```python
from build123d import *

# Parameters (mm, degrees)
SKETCH1_R           = 11
BOSS_EXTRUDE1_DEPTH = 20.45
SKETCH2_R           = 11
SKETCH2_R_2         = 10.8
CUT_EXTRUDE1_DEPTH  = 30.5
SKETCH5_R           = 0.8
CUT_EXTRUDE2_DEPTH  = 3
BOSS_EXTRUDE2_DEPTH = 2
SKETCH7_R           = 3
BOSS_EXTRUDE3_DEPTH = 12
CUT_EXTRUDE3_DEPTH  = 1
CIRPATTERN1_COUNT   = 4
CIRPATTERN2_COUNT   = 4
SKETCH11_R          = 5
BOSS_EXTRUDE4_DEPTH = 0.25
SKETCH12_R          = 11.05
BOSS_EXTRUDE5_DEPTH = 7
SKETCH14_R          = 1.0375
CUT_EXTRUDE4_DEPTH  = 3
SKETCH16_R          = 10.8
SKETCH16_R_2        = 10.3
CUT_EXTRUDE5_DEPTH  = 1.5
CUT_EXTRUDE6_DEPTH  = 0.5
CUT_EXTRUDE7_DEPTH  = 1.5
CHAMFER1_SIZE       = 0.25
CUT_EXTRUDE8_DEPTH  = 0.5
SKETCH20_R          = 0.5
BOSS_EXTRUDE7_DEPTH = 0.5
CIRPATTERN4_COUNT   = 2
SKETCH22_R          = 3
BOSS_EXTRUDE8_DEPTH = 2
SKETCH23_R          = 1
BOSS_EXTRUDE9_DEPTH = 9.2
CHAMFER2_SIZE       = 0.25
SKETCH24_R          = 1.552462654
CUT_EXTRUDE9_DEPTH  = 10
SKETCH25_R          = 3
CUT_EXTRUDE10_DEPTH = 8


with BuildPart() as part:
    # Sketch1 → Boss-Extrude1 (new body, symmetric)
    with BuildSketch(Plane.XY):
        Circle(SKETCH1_R)
    extrude(amount=BOSS_EXTRUDE1_DEPTH, both=True)

    # Sketch2 → Cut-Extrude1 (cut, through all)
    with BuildSketch(Plane(origin=(0, 0, 9.05), x_dir=(-1, 0, 0), z_dir=(0, 0, -1))):
        Circle(SKETCH2_R)
        Circle(SKETCH2_R_2, mode=Mode.SUBTRACT)
    extrude(amount=CUT_EXTRUDE1_DEPTH, mode=Mode.SUBTRACT)

    # Sketch5 → Cut-Extrude2 (cut)
    with BuildSketch(Plane.XY.offset(20.45)):
        with Locations((-6.363961031, 6.363961031)):
            Circle(SKETCH5_R)
        with Locations((6.363961031, 6.363961031)):
            Circle(SKETCH5_R)
        with Locations((6.363961031, -6.363961031)):
            Circle(SKETCH5_R)
        with Locations((-6.363961031, -6.363961031)):
            Circle(SKETCH5_R)
        with BuildLine():
            Line((-1.5, 9), (-1.5, 10.897247359))
            ThreePointArc((-1.5, 10.897247359), (0, 11), (1.5, 10.897247359))
            Line((1.5, 10.897247359), (1.5, 9))
            ThreePointArc((1.5, 9), (0, 7.5), (-1.5, 9))
        make_face()
        with BuildLine():
            Line((9, 1.5), (10.897247359, 1.5))
            ThreePointArc((10.897247359, 1.5), (11, 0), (10.897247359, -1.5))
            Line((10.897247359, -1.5), (9, -1.5))
            ThreePointArc((9, -1.5), (7.5, 0), (9, 1.5))
        make_face()
        with BuildLine():
            Line((1.5, -9), (1.5, -10.897247359))
            ThreePointArc((1.5, -10.897247359), (0, -11), (-1.5, -10.897247359))
            Line((-1.5, -10.897247359), (-1.5, -9))
            ThreePointArc((-1.5, -9), (0, -7.5), (1.5, -9))
        make_face()
        with BuildLine():
            Line((-9, -1.5), (-10.897247359, -1.5))
            ThreePointArc((-10.897247359, -1.5), (-11, 0), (-10.897247359, 1.5))
            Line((-10.897247359, 1.5), (-9, 1.5))
            ThreePointArc((-9, 1.5), (-7.5, 0), (-9, -1.5))
        make_face()
    extrude(amount=-CUT_EXTRUDE2_DEPTH, mode=Mode.SUBTRACT)

    # Sketch3 → Cut-Revolve3 (revolve, cut)
    with BuildSketch(Plane(origin=(0, 0, 0), x_dir=(0, 0, -1), z_dir=(1, 0, 0))):
        with BuildLine():
            ThreePointArc((-9.05, 10.4), (-8.932842712, 10.682842712), (-8.65, 10.8))
            Line((-8.65, 10.8), (-9.05, 10.8))
            Line((-9.05, 10.8), (-9.05, 10.4))
        make_face()
    revolve(axis=Axis((0, 0, -27.758521673), (0, 0, 1)), mode=Mode.SUBTRACT)

    # Sketch6 → Boss-Extrude2 (add)
    with BuildSketch(Plane.XY.offset(20.45)):
        with BuildLine():
            Line((-6, -3.605551275), (-6, 3.605551275))
            ThreePointArc((-6, 3.605551275), (0, 7), (6, 3.605551275))
            Line((6, 3.605551275), (6, -3.605551275))
            ThreePointArc((6, -3.605551275), (0, -7), (-6, -3.605551275))
        make_face()
    extrude(amount=BOSS_EXTRUDE2_DEPTH)

    # Sketch7 → Boss-Extrude3 (add)
    with BuildSketch(Plane.XY.offset(22.45)):
        Circle(SKETCH7_R)
    extrude(amount=BOSS_EXTRUDE3_DEPTH)

    # Sketch9 → Revolve1 (revolve)
    with BuildSketch(Plane(origin=(0, 9, 0), x_dir=(1, 0, 0), z_dir=(0, 1, 0))):
        with BuildLine():
            Line((0, -17.45), (0, -18.65))
            Line((0, -18.65), (0.85, -18.65))
            ThreePointArc((0.85, -18.65), (1.168198052, -18.518198052), (1.3, -18.2))
            Line((1.3, -18.2), (1.3, -17.45))
            Line((1.3, -17.45), (0, -17.45))
        make_face()
    revolve1 = revolve(axis=Axis((0, 9, 17.45), (0, 0, 1)))

    # Sketch10 → Cut-Extrude3 (cut)
    with BuildSketch(Plane.XY.offset(18.65)):
        with BuildLine():
            Line((0.15, 9.15), (1.291317157, 9.15))
            ThreePointArc((1.291317157, 9.15), (1.3, 9), (1.291317157, 8.85))
            Line((1.291317157, 8.85), (0.15, 8.85))
            Line((0.15, 8.85), (-0.15, 8.85))
            Line((-0.15, 8.85), (-1.291317157, 8.85))
            ThreePointArc((-1.291317157, 8.85), (-1.3, 9), (-1.291317157, 9.15))
            Line((-1.291317157, 9.15), (-0.15, 9.15))
            Line((-0.15, 9.15), (0.15, 9.15))
        make_face()
    cut_extrude3 = extrude(amount=-CUT_EXTRUDE3_DEPTH, mode=Mode.SUBTRACT)

    # CirPattern1: Revolve1 ×4 about axis
    cirpattern1_axis = Axis((0, 0, 0), (0, 0, 1))
    for i in range(1, CIRPATTERN1_COUNT):
        add(revolve1.rotate(cirpattern1_axis, i * 360 / CIRPATTERN1_COUNT))

    # CirPattern2: Cut-Extrude3 ×4 about axis
    cirpattern2_axis = Axis((0, 0, -27.758521673), (0, 0, 1))
    for i in range(1, CIRPATTERN2_COUNT):
        add(cut_extrude3.rotate(cirpattern2_axis, i * 360 / CIRPATTERN2_COUNT), mode=Mode.SUBTRACT)

    # Sketch11 → Boss-Extrude4 (add)
    with BuildSketch(Plane.XY.offset(22.45)):
        Circle(SKETCH11_R)
    extrude(amount=BOSS_EXTRUDE4_DEPTH)

    # Sketch12 → Boss-Extrude5 (add, symmetric)
    with BuildSketch(Plane(origin=(0, 0, 19.75), x_dir=(-1, 0, 0), z_dir=(0, 0, -1))):
        Circle(SKETCH12_R)
    extrude(amount=BOSS_EXTRUDE5_DEPTH, both=True)

    # Sketch14 → Cut-Extrude4 (cut, symmetric)
    with BuildSketch(Plane(origin=(0, 0, 0), x_dir=(0, 0, -1), z_dir=(1, 0, 0))):
        with Locations((-30.35, 0)):
            Circle(SKETCH14_R)
    extrude(amount=CUT_EXTRUDE4_DEPTH, both=True, mode=Mode.SUBTRACT)

    # Sketch16 → Cut-Extrude5 (cut)
    with BuildSketch(Plane(origin=(0, 0, -20.45), x_dir=(-1, 0, 0), z_dir=(0, 0, -1))):
        Circle(SKETCH16_R)
        Circle(SKETCH16_R_2, mode=Mode.SUBTRACT)
    extrude(amount=-CUT_EXTRUDE5_DEPTH, mode=Mode.SUBTRACT)

    # Sketch17 → Cut-Extrude6 (cut)
    with BuildSketch(Plane(origin=(0, 0, -20.45), x_dir=(-1, 0, 0), z_dir=(0, 0, -1))):
        with BuildLine():
            Line((0, 8), (-1, 8))
            Line((-1, 8), (-1, 10.251341376))
            ThreePointArc((-1, 10.251341376), (0, 10.3), (1, 10.251341376))
            Line((1, 10.251341376), (1, 8))
            Line((1, 8), (0, 8))
        make_face()
        with BuildLine():
            Line((8, 1), (10.251341376, 1))
            ThreePointArc((10.251341376, 1), (10.3, 0), (10.251341376, -1))
            Line((10.251341376, -1), (8, -1))
            Line((8, -1), (8, 0))
            Line((8, 0), (8, 1))
        make_face()
        with BuildLine():
            Line((1, -8), (1, -10.251341376))
            ThreePointArc((1, -10.251341376), (0, -10.3), (-1, -10.251341376))
            Line((-1, -10.251341376), (-1, -8))
            Line((-1, -8), (0, -8))
            Line((0, -8), (1, -8))
        make_face()
        with BuildLine():
            Line((-8, -1), (-10.251341376, -1))
            ThreePointArc((-10.251341376, -1), (-10.3, 0), (-10.251341376, 1))
            Line((-10.251341376, 1), (-8, 1))
            Line((-8, 1), (-8, 0))
            Line((-8, 0), (-8, -1))
        make_face()
    extrude(amount=-CUT_EXTRUDE6_DEPTH, mode=Mode.SUBTRACT)

    # Sketch18 → Cut-Extrude7 (cut)
    with BuildSketch(Plane(origin=(0, 0, -20.45), x_dir=(-1, 0, 0), z_dir=(0, 0, -1))):
        with BuildLine():
            Line((-1, 10.251341376), (-1, 9.447221814))
            ThreePointArc((-1, 9.447221814), (0, 9.5), (1, 9.447221814))
            Line((1, 9.447221814), (1, 10.251341376))
            ThreePointArc((1, 10.251341376), (0, 10.3), (-1, 10.251341376))
        make_face()
        with BuildLine():
            Line((10.251341376, 1), (9.447221814, 1))
            ThreePointArc((9.447221814, 1), (9.5, 0), (9.447221814, -1))
            Line((9.447221814, -1), (10.251341376, -1))
            ThreePointArc((10.251341376, -1), (10.3, 0), (10.251341376, 1))
        make_face()
        with BuildLine():
            Line((1, -10.251341376), (1, -9.447221814))
            ThreePointArc((1, -9.447221814), (0, -9.5), (-1, -9.447221814))
            Line((-1, -9.447221814), (-1, -10.251341376))
            ThreePointArc((-1, -10.251341376), (0, -10.3), (1, -10.251341376))
        make_face()
        with BuildLine():
            Line((-10.251341376, -1), (-9.447221814, -1))
            ThreePointArc((-9.447221814, -1), (-9.5, 0), (-9.447221814, 1))
            Line((-9.447221814, 1), (-10.251341376, 1))
            ThreePointArc((-10.251341376, 1), (-10.3, 0), (-10.251341376, -1))
        make_face()
    extrude(amount=-CUT_EXTRUDE7_DEPTH, mode=Mode.SUBTRACT)

    # Chamfer1
    chamfer1_edges = [part.edges().sort_by_distance(p)[0] for p in [
        (-7.283199846, 7.283199846, -20.45),
        (7.283199846, 7.283199846, -20.45),
        (7.283199846, -7.283199846, -20.45),
        (-7.283199846, -7.283199846, -20.45),
    ]]
    chamfer(chamfer1_edges, length=CHAMFER1_SIZE)

    # Sketch19 → Cut-Extrude8 (cut)
    with BuildSketch(Plane(origin=(0, 0, -20.45), x_dir=(-1, 0, 0), z_dir=(0, 0, -1))):
        with BuildLine():
            Line((-6.545347941, 4.777580988), (-8.313114894, 6.545347941))
            ThreePointArc((-8.313114894, 6.545347941), (-7.481626123, 7.481626123), (-6.545347941, 8.313114894))
            Line((-6.545347941, 8.313114894), (-4.777580988, 6.545347941))
            Line((-4.777580988, 6.545347941), (-6.545347941, 4.777580988))
        make_face()
        with BuildLine():
            Line((4.777580988, -6.545347941), (6.545347941, -8.313114894))
            ThreePointArc((6.545347941, -8.313114894), (7.481626123, -7.481626123), (8.313114894, -6.545347941))
            Line((8.313114894, -6.545347941), (6.545347941, -4.777580988))
            Line((6.545347941, -4.777580988), (4.777580988, -6.545347941))
        make_face()
    extrude(amount=-CUT_EXTRUDE8_DEPTH, mode=Mode.SUBTRACT)

    # Sketch20 → Boss-Extrude7 (add)
    with BuildSketch(Plane(origin=(5.661464464, 5.661464464, 0), x_dir=(0, 0, -1), z_dir=(0.707106781, 0.707106781, 0))):
        with BuildLine():
            Line((19.95, 1.25), (25.45, 1.25))
            ThreePointArc((25.45, 1.25), (26.7, 0), (25.45, -1.25))
            Line((25.45, -1.25), (19.95, -1.25))
            Line((19.95, -1.25), (19.95, 1.25))
        make_face()
        with Locations((25.45, 0)):
            Circle(SKETCH20_R, mode=Mode.SUBTRACT)
    boss_extrude7 = extrude(amount=BOSS_EXTRUDE7_DEPTH)

    # CirPattern4: Boss-Extrude7 ×2 about axis
    cirpattern4_axis = Axis((0, 0, 0), (0, 0, 1))
    for i in range(1, CIRPATTERN4_COUNT):
        add(boss_extrude7.rotate(cirpattern4_axis, i * 360 / CIRPATTERN4_COUNT))

    # Sketch22 → Boss-Extrude8 (add)
    with BuildSketch(Plane(origin=(0, 0, -20.45), x_dir=(-1, 0, 0), z_dir=(0, 0, -1))):
        Circle(SKETCH22_R)
    extrude(amount=BOSS_EXTRUDE8_DEPTH)

    # Sketch23 → Boss-Extrude9 (add)
    with BuildSketch(Plane(origin=(0, 0, -22.45), x_dir=(-1, 0, 0), z_dir=(0, 0, -1))):
        Circle(SKETCH23_R)
    extrude(amount=BOSS_EXTRUDE9_DEPTH)

    # Chamfer2
    chamfer2_edges = [part.edges().sort_by_distance(p)[0] for p in [
        (3, 0, -22.45),
    ]]
    chamfer(chamfer2_edges, length=CHAMFER2_SIZE)

    # Sketch24 → Cut-Extrude9 (cut)
    with BuildSketch(Plane(origin=(0, 0, -31.65), x_dir=(-1, 0, 0), z_dir=(0, 0, -1))):
        Circle(SKETCH24_R)
    extrude(amount=-CUT_EXTRUDE9_DEPTH, mode=Mode.SUBTRACT)

    # Sketch25 → Cut-Extrude10 (cut)
    with BuildSketch(Plane.XY.offset(34.45)):
        Circle(SKETCH25_R)
    extrude(amount=-CUT_EXTRUDE10_DEPTH, mode=Mode.SUBTRACT)


solid = part.part
```
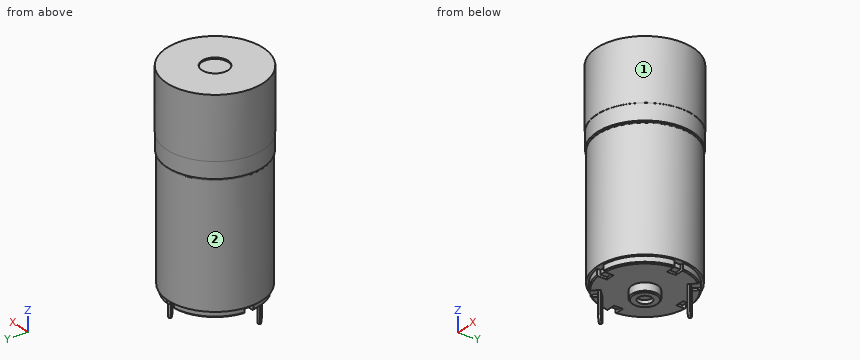
Model file for the job. Use its own axes, mm. Face numbers are marked on the shaded views. A direction names the side the tool comes from. Round coordinates to 2 decimals unless told otherwise and drop trailing zeros. Write each loop counter-clockwise with the first axis right and the second up, starting at its lowest first coordinate (ties: lowest second). Pieces come first, ordered by that corner, then holes. Notation, with made-up numbers: M 13,-16 L 45,-16 A10 cw 45,-3 Z; hole C -31,20.25 d8. An arc over 180 degrees is marked long. Put each result on its own line as item: value.
Item 1: Cut at A-A (z = 19). List the corners of the cut face in (x, y).
Responses:
outline: C 0,0 d22.1
Item 2: Tool access for the marked faces 1 and 2: list every direction of +Z, -Z, +X, -X, +Y, -Y with a clear straight run to the whole face (end or side of a thin tool).
Responses:
face 1: +Z, -Z
face 2: -Z
Item 3: Flat gauge pins, fed straight in: P1, Ø1.5, axis at x = -3.5, z = -12.5, coming from the -Y side; P2, Ø0.8, axis at y = -9.5, z = -19.5, coming from the -X side; P3, Ø8, axis at x = 6, z = 3.5, coming from the -Y side. Where does each tip first touch, or does it go through?
Responses:
P1: y = -10.44
P2: x = -4.82
P3: y = -10.61
Item 4: Probe L1, parallel to Y at x = 0, z = -22.1; L2, parallel to Z at x = -4.5, y = 3; L3, parallel to Z at x = 3.75, y = 10.25. List the from-to ranges inside material, lowest first. Write a range as from..to.
Responses:
L1: -3..-1.55, 1.55..3
L2: -20.45..26.75
L3: 9.05..26.75
